Print and shaded views of the part. All mm, measured from the part's lowest x, y and z. A direction names the side the tool comes from. Round coordinates to 2 decimals unless told otherwise and drop trailing zeros. Loops run counter-clockwise (first coordinate to the right, second up) from the corner with the lowest first, then second, coordinate; pieces in that order, holes last. Notation, with made-up numbers: (-14.75, 81) - (28.25, 81) arc R19 cw to (28.25, 97) - close; hole circle Ø1 at (52.25, 19.5). An arc over 180 degrees is marked (long way). Use one line per item in the form item = value. Start each with the question number.
Q1. Saw through at C-C (z = 21.25). Give the cut face in (x, y) (1 decimal), then the cut area to 3 significant figures.
Q2. Pin check, flat tips, straight feed: pin 1 (6 mm diameter, centred on y = 39.5, z = 6.5, fed in from +X); pin 2 (1.5 mm diameter, centred on x = 28, z = 9.5, fed in from +Y); pin 3 (5 mm diameter, centred on x = 24.5, z = 9, fed in from +Y). Stop position of each tip, or through.
Q3. Saw through at A-A (y = 37). Give the cut face in (x, z).
Q4. Mould opens along Y. For the marked faces 3, 4 and 5 say: released by +Y, released by -Y, zero draft, split by the parting line, or undercut.
Q5. Saw through at D-D (x = 5). Give the cut face in (y, z).
Q6. 3-axis set-ups, long thin cutter, end or side, ignore diameter. For the marked faces 1 and 2: which of +Z, -Z, +X, -X, +Y, -Y reach the whole face in a straight line?
Q7. Saw through at B-B (x = 16). Give the cut face in (y, z) (1 decimal).
Q8. Drill centre lines: line 1 (Y direction, x = 20, z = 22.5) (1 decimal); line 2 (Y direction, x = 18, z = 15) (1 decimal); line 3 (X direction, y = 28.5, z = 3.25) (1 decimal). Where is each one in solid material? Low to high.
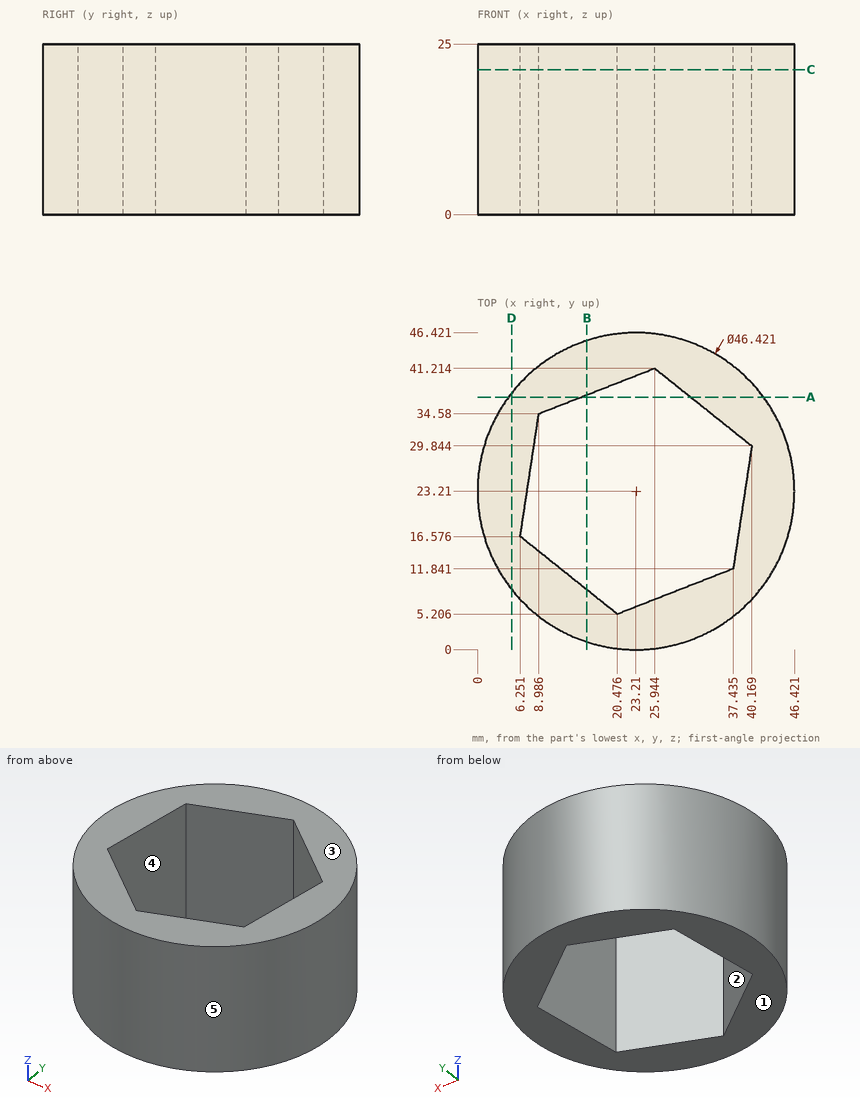
Report:
q1.outline = circle Ø46.4 at (23.2, 23.2); hole (6.3, 16.6) - (20.5, 5.2) - (37.4, 11.8) - (40.2, 29.8) - (25.9, 41.2) - (9, 34.6) - close
q1.area = 831 mm²
q2.pin_1 = 42.24
q2.pin_2 = 46.07
q2.pin_3 = 46.42
q3.outline = (4.54, 0) - (15.17, 0) - (15.17, 25) - (4.54, 25) - close; (31.22, 0) - (41.88, 0) - (41.88, 25) - (31.22, 25) - close
q4.face_3 = zero draft
q4.face_4 = undercut
q4.face_5 = split by the parting line
q5.outline = (8.82, 0) - (37.6, 0) - (37.6, 25) - (8.82, 25) - close
q6.face_1 = -Z, +X, -X, +Y, -Y
q6.face_2 = +Z, -Z
q7.outline = (1.1, 0) - (8.8, 0) - (8.8, 25) - (1.1, 25) - close; (37.3, 0) - (45.3, 0) - (45.3, 25) - (37.3, 25) - close
q8.line_1 = 0.2 to 5.6, 38.9 to 46.2
q8.line_2 = 0.6 to 7.2, 38.1 to 45.8
q8.line_3 = 0.6 to 8.1, 40 to 45.8
